Model file for the job. Use its own axes, mm. A direction names the side the tool comes from. Round coordinates to 2 decimals unless told otherwise and drop trailing zeros. Loops run counter-clockwise (first coordinate to the right, second up) from the corner with the lowest first, then second, coordinate; pieces in that order, holes last. Notation, with made-up numbers: M -2.75,74 L 3.25,74 A11 cw 3.25,85 Z; hole C -22.75,16 d11. An arc over 180 degrees is marked long. Use a Markdown table: item, result. Add a question column.
Item 1: Pin check, flat tips, straight feed: P1, Ø1.5, axis at x = 7.5, y = 4, coming from the +Z side; P2, Ø1.5, axis at x = 5, y = 8, coming from the +Z side. Stop position of each tip, or through.
Item 2: Saw through at B-B on y = 3. Write the cut outline in (x, z), then the cut area to 3 significant figures.
Item 3: Saw through at A-A on z = 0. Write the cut outline in (x, y).
Item 4: Tool access for faces 1 (the cylindrical face through (-0.715, 7.479, -7.125)), 2 (the cylindrical face through (1.802, 4.444, 5.723)): list every direction of +Z, -Z, +X, -X, +Y, -Y with a clear straight run to the whole face (end or side of a thin tool).
Item 5: Wall check: L1, parallel to Z at x = -0.25, y = 7.5; L2, parallel to X at y = 2.5, z = 0; L3, parallel to Y at x = 0, z = 9 (3 decimals). Give the ranges that are in metal, low to high. Write a range as from..to.
Item 6: Two-plate mould, pull along X, no slides. Class faces 3 (the flat face through (-5, 9, 5)), 4 (the cylindrical face through (-0.22, 3.5, 9.25)), 5 (the cylindrical face through (3.755, 4.444, 11.923)): +X half, -X half, draft (parallel to the pull), parting line (faces both ways), or undercut.
Item 7: Saw through at C-C on y = 4.5. Write the cut outline in (x, z) (3 decimals), then the cut area to 3 significant figures.
```python
from build123d import *

# Parameters (mm, degrees)
SKETCH1_R                      = 12.5
SKETCH1_R_2                    = 6
BOSS_EXTRUDE1_DEPTH            = 9
CHAMFER1_SIZE                  = 0.5
M2_5X0_45_TAPPED_HOLE1_REACH   = 31.364
M2_5X0_45_TAPPED_HOLE1_BORE_R  = 1.025
F_3_1_3_1_DIAMETER_HOLE1_D     = 3.1
F_3_1_3_1_DIAMETER_HOLE1_DEPTH = 3
F_3_1_3_1_DIAMETER_HOLE1_TIP   = 0.931333959


with BuildPart() as part:
    # Sketch1 → Boss-Extrude1 (new body)
    with BuildSketch(Plane(origin=(0, 0, 0), x_dir=(1, 0, 0), z_dir=(0, 1, 0))):
        with Locations(Location((0, 0, 0), (0, 0, 270))):
            Circle(SKETCH1_R)
        with Locations(Location((0, 0, 0), (0, 0, 270))):
            Circle(SKETCH1_R_2, mode=Mode.SUBTRACT)
    extrude(amount=BOSS_EXTRUDE1_DEPTH)

    # Chamfer1
    chamfer1_edges = [part.edges().sort_by_distance(p)[0] for p in [
        (0, 0, -12.5),
        (0, 9, -12.5),
        (0, 0, -6),
        (0, 9, -6),
    ]]
    chamfer(chamfer1_edges, length=CHAMFER1_SIZE)

    # M2.5x0.45 Tapped Hole1 bore → M2.5x0.45 Tapped Hole1 (cut, up to next)
    with BuildSketch(Plane.XY.offset(12.5), mode=Mode.PRIVATE) as m2_5x0_45_tapped_hole1_sk1:
        with Locations((0, 4.5)):
            Circle(M2_5X0_45_TAPPED_HOLE1_BORE_R)
    m2_5x0_45_tapped_hole1_tool1 = extrude(m2_5x0_45_tapped_hole1_sk1.sketch, amount=-M2_5X0_45_TAPPED_HOLE1_REACH, mode=Mode.PRIVATE) & part.part
    add(m2_5x0_45_tapped_hole1_tool1.solids().sort_by_distance((0, 4.5, 12.5))[0], mode=Mode.SUBTRACT)

    # Ø3.1 (3.1) Diameter Hole1
    with Locations(Plane(origin=(0, 9, 0), x_dir=(1, 0, 0), z_dir=(0, 1, 0))):
        with Locations((0, 8.5)):
            Hole(F_3_1_3_1_DIAMETER_HOLE1_D / 2, depth=F_3_1_3_1_DIAMETER_HOLE1_DEPTH)
            with Locations((0, 0, -(F_3_1_3_1_DIAMETER_HOLE1_DEPTH + F_3_1_3_1_DIAMETER_HOLE1_TIP / 2))):  # 118° drill point
                Cone(0, F_3_1_3_1_DIAMETER_HOLE1_D / 2, F_3_1_3_1_DIAMETER_HOLE1_TIP, mode=Mode.SUBTRACT)


solid = part.part
```
Entries:
| question | item | result |
|---|---|---|
| 1 | P1 | z = 10.52 |
| 1 | P2 | z = 11.76 |
| 2 | outline | C 0,0 d25; hole C 0,0 d12 |
| 2 | area | 378 mm2 |
| 3 | outline | M -12.5,0.5 L -12,0 L -6.5,0 L -6,0.5 L -6,8.5 L -6.5,9 L -12,9 L -12.5,8.5 Z; M 6,0.5 L 6.5,0 L 12,0 L 12.5,0.5 L 12.5,8.5 L 12,9 L 6.5,9 L 6,8.5 Z |
| 4 | face 1 | +Y |
| 4 | face 2 | +Y, -Y |
| 5 | L1 | -12.5..-10.03, -6.97..-5.99, 5.99..12.5 |
| 5 | L2 | -12.5..-6, 6..12.5 |
| 5 | L3 | 0..3.475, 5.525..9 |
| 6 | face 3 | draft |
| 6 | face 4 | undercut |
| 6 | face 5 | parting line |
| 7 | outline | M -1.025,5.912 L -1.025,12.458 A12.5 ccw long 1.025,12.458 L 1.025,5.912 A6 cw long Z |
| 7 | area | 364 mm2 |
